The listing builds one solid part. Answer for the finished solid, in the listing's coordinates (mm). A direction names the side the tool comes from. Give positions to 0.01 mm unless a question says otherwise; leave off trailing zeros. Loops run counter-clockwise (first coordinate to the right, second up) from the corner with the lowest first, then second, coordinate; pieces in that order, holes last. Notation, with made-up numbers: (17.25, 64.25) - (63.25, 64.25) arc R18 cw to (63.25, 86.25) - close; hole circle Ø6 at (-36, 73). An arc over 180 degrees is marked (long way). Answer as CSV lines item,"result". Start each with the question number.
1) A cutting plane is placed at C-C (y = -79). Determine the outline of the cut face in (x, z).
2) Find the intervals of material crossed by line 1 along Y through (x, z) = (-207.5, 12.5); line 2 along Y through (x, z) = (-178, 15); line 3 along X through (y, z) = (43, 15.5), in increasing order.
3) For a pull along X with two mould halves and no side action, classify faces 1 (the face through (-310.658, 6, 20)), 2 (the face through (-201, 109, 40)), 3 (the face through (-290.658, -2, 20)) as pulls with the +X half, pulls with the -X half, needs draft (parallel to the pull), parting line crosses it, or undercut.
4) A cutting plane is placed at B-B (y = 101). Determine the outline of the cut face in (x, z).
5) A cutting plane is placed at D-D (x = -80). Determine the outline of the cut face in (y, z), and give its area (3 significant figures).
6) A cutting plane is placed at A-A (z = 15.5). Determine the outline of the cut face in (x, y), and give its area (3 significant figures).
7) Flat-ended cylindrical pins translate along their axes: pin 1 (1.5 mm diameter, centred on y = 109.5, z = 30.5, fed in from +X); pin 2 (1 mm diameter, centred on x = -86.5, z = 26, fed in from -Y); pin 3 (2 mm diameter, centred on y = -24.5, z = 36, fed in from +X). Find the tip coordinate at first contact, or state that the pin passes through.
8) For faces 4 (the face through (-233, -135.32, 20)), 5 (the face through (-192, 104.68, 20)), determine the directions among +Z, -Z, +X, -X, +Y, -Y from which every point of the face is accessible in a straight line to the end or side of a thin tool.
```python
from build123d import *

# Parameters (mm, degrees)
BOSS_EXTRUDE2_DEPTH = 40
FILLET3_R           = 20
SKETCH2_R           = 2.5
CUT_EXTRUDE1_DEPTH  = 10


with BuildPart() as part:
    # Sketch1 → Boss-Extrude2 (new body)
    with BuildSketch(Plane.XY):
        Polygon((-310.658255987, -135.320069059), (-160.658255987, -135.320069059), (-42.316331357, 144.679930941), (-310.658255987, 144.679930941), align=None)
        Polygon((-290.658255987, 104.679930941), (-80.935291782, 104.679930941), (-169.691735254, -105.320069059), (-290.658255987, -105.320069059), align=None, mode=Mode.SUBTRACT)
    extrude(amount=BOSS_EXTRUDE2_DEPTH)

    # Fillet3
    fillet3_edges = [part.edges().sort_by_distance(p)[0] for p in [
        (-80.935291782, 104.679930941, 20),
        (-290.658255987, 104.679930941, 20),
        (-290.658255987, -105.320069059, 20),
        (-169.691735254, -105.320069059, 20),
        (-42.316331357, 144.679930941, 20),
        (-160.658255987, -135.320069059, 20),
        (-310.658255987, -135.320069059, 20),
        (-310.658255987, 144.679930941, 20),
    ]]
    fillet(fillet3_edges, radius=FILLET3_R)

    # Sketch2 → Cut-Extrude1 (cut)
    with BuildSketch(Plane.XY.offset(40)):
        with Locations((-250.658255987, 137.179930941)):
            Circle(SKETCH2_R)
        with Locations((-210.658255987, 137.179930941)):
            Circle(SKETCH2_R)
        with Locations((-230.658255987, 122.179930941)):
            Circle(SKETCH2_R)
    cut_extrude1 = extrude(amount=-CUT_EXTRUDE1_DEPTH, mode=Mode.SUBTRACT)

    # Mirror1: Cut-Extrude1 across plane
    add(cut_extrude1.mirror(Plane.ZY.offset(175.658255987)), mode=Mode.SUBTRACT)


solid = part.part
```
Ans:
1,outline,"(-310.66, 0) - (-290.66, 0) - (-290.66, 40) - (-310.66, 40) - close; (-158.57, 0) - (-136.85, 0) - (-136.85, 40) - (-158.57, 40) - close"
2,line 1,"-135.32 to -105.32, 104.68 to 144.68"
2,line 2,"-135.32 to -104.7, 104.68 to 144.68"
2,line 3,"-310.66 to -290.66, -107 to -85.29"
3,face 1,"pulls with the -X half"
3,face 2,"needs draft"
3,face 3,"undercut"
4,outline,"(-310.66, 0) - (-282.22, 0) - (-282.22, 40) - (-310.66, 40) - close; (-99.54, 0) - (-60.78, 0) - (-60.78, 40) - (-99.54, 40) - close"
5,outline,"(55.52, 0) - (144.68, 0) - (144.68, 40) - (55.52, 40) - close"
5,area,"3,570 mm2"
6,outline,"(-310.66, -115.32) arc R20 ccw to (-290.66, -135.32) - (-173.92, -135.32) arc R20 ccw to (-155.5, -123.11) - (-54.06, 116.89) arc R20 ccw to (-72.48, 144.68) - (-290.66, 144.68) arc R20 ccw to (-310.66, 124.68) - close; hole (-290.66, -85.32) arc R20 ccw to (-270.66, -105.32) - (-182.95, -105.32) arc R20 ccw to (-164.53, -93.11) - (-92.68, 76.89) arc R20 ccw to (-111.1, 104.68) - (-270.66, 104.68) arc R20 ccw to (-290.66, 84.68) - close"
6,area,"23,800 mm2"
7,pin 1,"x = -56.87"
7,pin 2,"y = 38.96"
7,pin 3,"x = -113.4"
8,face 4,"+Z, -Z, +X, -X, -Y"
8,face 5,"+Z, -Z"
